The drawing under review shows one solid part. Ordinate dimensions are in mm from its lowest x, y, z. A direction names the side the tool comes from. Coordinates: 2 decimals unless noted, no trailing zeros. Loops run counter-clockwise (first coordinate to the right, second up) from the corner with the lowest first, then second, coordinate; pieces in that order, holes last.
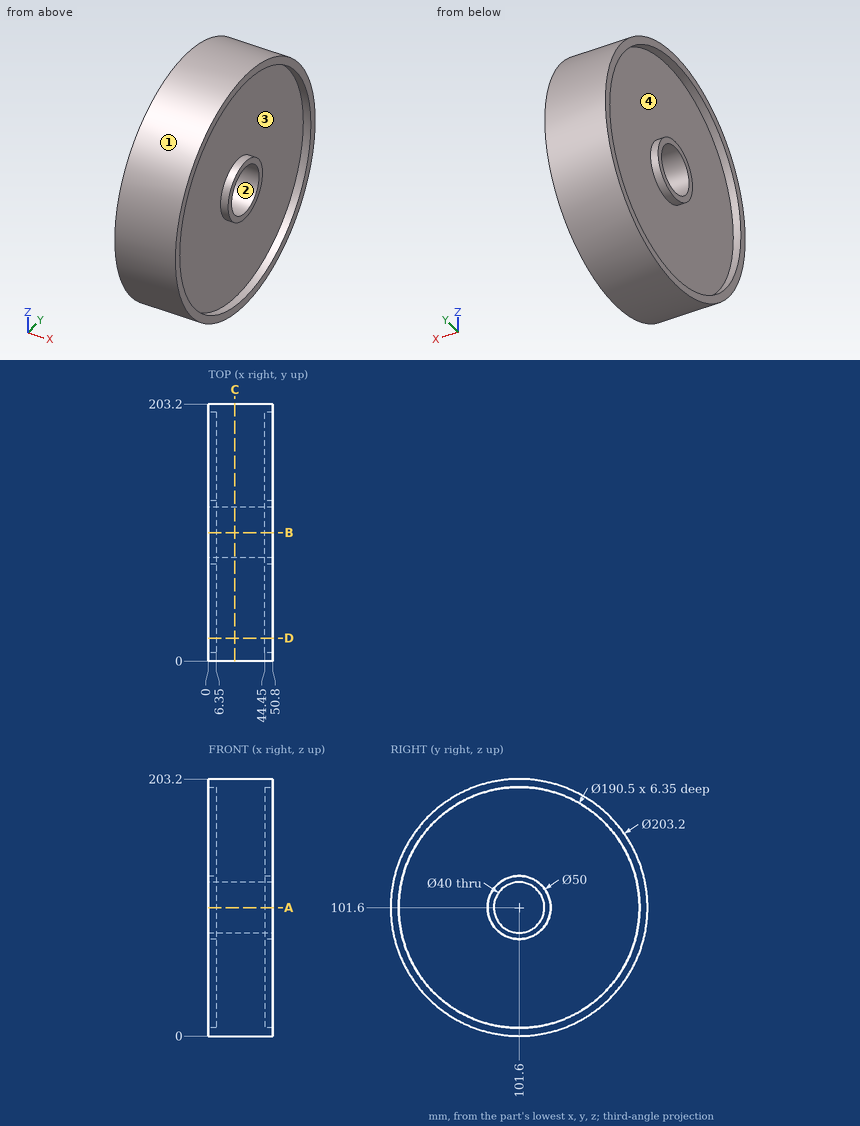
Q1. For line 1 (Y direction, x = 47, z = 101.6); line 2 (Z direction, x = 48, y = 101); line 3 (Z direction, x = 21, y = 101), list the stretches that pass through material, from the lowest coordinate up.
Q2. Clearance check with flat-ended pins moving along their axes: pin 1 Ø1.5 at (x, y) = (38, 42) entering from +Z; pin 2 Ø3 at (x, z) = (24, 179) entering from -Y; pin 3 Ø2 at (x, z) = (25.5, 154.5) entering from +Y. State where each tip first meets the part, or that it passes through.
Q3. Take a section at A-A, the plane z = 101.6. Write out the cut boundary in (x, y), then the cut area to 3 significant figures.
Q4. Machinability: for the marked faces 3 and 4, which of the approach directions +Z, -Z, +X, -X, +Y, -Y give a long, thin tool a straight path to every point of the face, cutting with its end or side? Answer none if there is none.
Q5. Take a section at C-C, the plane x = 21. Write out the cut boundary in (y, z).
Q6. The part is to be moulded in two halves that separate along Z. For the marked faces 1 and 2, say which applies: pulls with the +Z half, pulls with the -Z half, needs draft (parallel to the pull), parting line crosses it, or undercut.
Q7. Take a section at D-D, the plane y = 18. Write out the cut boundary in (x, z).
Entries:
1. line 1: y = 0 to 6.35, 76.6 to 81.6, 121.6 to 126.6, 196.85 to 203.2
1. line 2: z = 0 to 6.35, 76.61 to 81.61, 121.59 to 126.59, 196.85 to 203.2
1. line 3: z = 0 to 81.61, 121.59 to 203.2
2. pin 1: stops at z = 184.42
2. pin 2: stops at y = 34.06
2. pin 3: stops at y = 188.94
3. outline: (0, 0) - (50.8, 0) - (50.8, 6.35) - (44.45, 6.35) - (44.45, 76.6) - (50.8, 76.6) - (50.8, 81.6) - (0, 81.6) - (0, 76.6) - (6.35, 76.6) - (6.35, 6.35) - (0, 6.35) - close; (0, 121.6) - (50.8, 121.6) - (50.8, 126.6) - (44.45, 126.6) - (44.45, 196.85) - (50.8, 196.85) - (50.8, 203.2) - (0, 203.2) - (0, 196.85) - (6.35, 196.85) - (6.35, 126.6) - (0, 126.6) - close
3. area: 6,510 mm2
4. face 3: +X
4. face 4: -X
5. outline: circle Ø203.2 at (101.6, 101.6); hole circle Ø40 at (101.6, 101.6)
6. face 1: parting line crosses it
6. face 2: undercut
7. outline: (0, 43.86) - (50.8, 43.86) - (50.8, 55.95) - (44.45, 55.95) - (44.45, 147.25) - (50.8, 147.25) - (50.8, 159.34) - (0, 159.34) - (0, 147.25) - (6.35, 147.25) - (6.35, 55.95) - (0, 55.95) - close
